Job drawing, mm, ordinate dimensions from the low corner. One solid piece. A direction names the side the tool comes from. Give positions to 0.01 mm unless a question says otherwise; leave off trailing zeros. Order: outer loops, then holes, each group sorted by start corner. A loop starts at its lowest first (then second) coordinate and runs counter-clockwise, first axis right, second up. Notation, with made-up numbers: (70.25, -36.5) - (101.25, -36.5) arc R32 cw to (101.25, -0.5) - close; hole circle Ø10 at (44.25, 56.25). An arc over 180 degrees is marked (long way). Use a Markdown table: item, result. Add a question column.
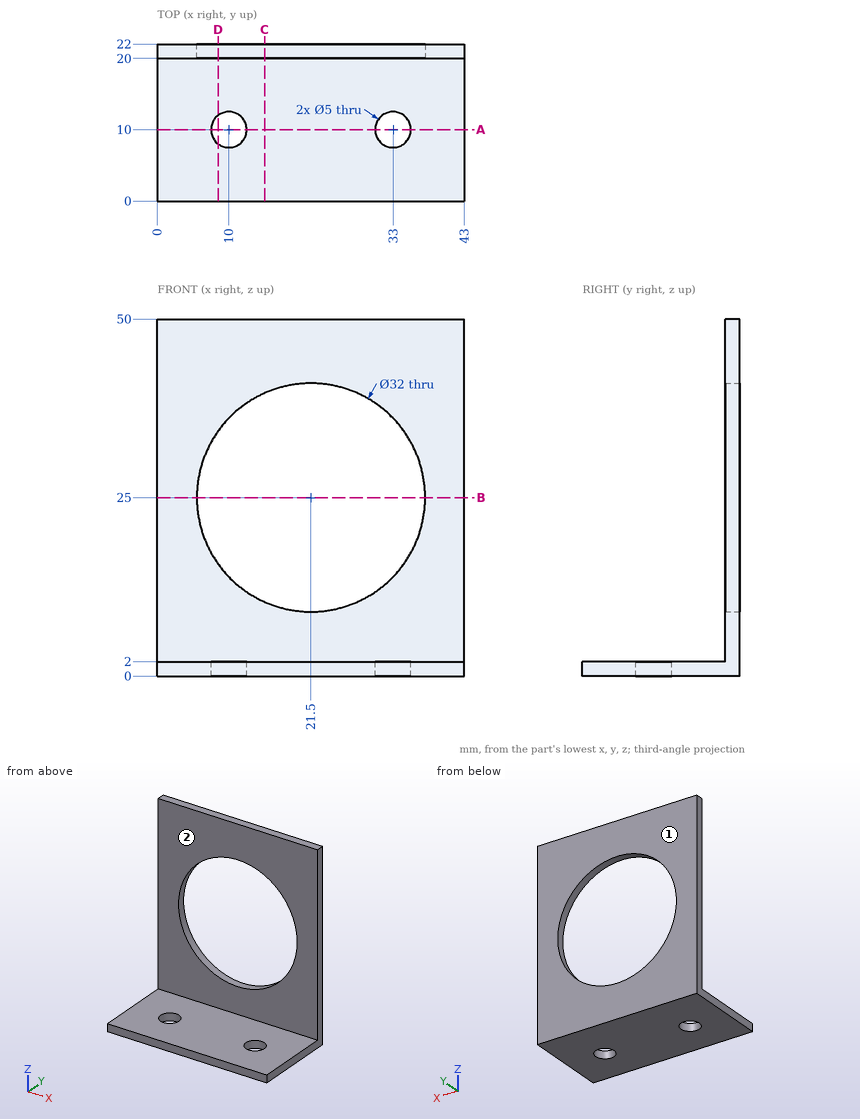
1. Tool access for the marked faces 1 and 2: list every direction of +Z, -Z, +X, -X, +Y, -Y with a clear straight run to the whole face (end or side of a thin tool).
2. Pin check, flat tips, straight feed: P1, Ø8, axis at x = 33, y = 10, coming from the +Z side; P2, Ø4.5, axis at x = 10, y = 10, coming from the -Z side. Stop position of each tip, or through.
3. Drill centre lines: probe 1 along X at (y, z) = (10, 0.6); probe 2 along Z at (x, y) = (21.5, 20.6); probe 3 along Y at (x, z) = (33, 0.7). Where is each one in solid material? Low to high. Write a range as [from, to].
4. Cut at B-B (z = 25). Write the cut outline in (x, y), plus the area to 3 significant figures.
5. Cut at C-C (x = 15). Write the cut outline in (y, z), plus the area to 3 significant figures.
6. Cut at D-D (x = 8.5). Write the cut outline in (y, z).
7. Cut at A-A (y = 10). Write the cut outline in (x, z), plus the area to 3 significant figures.
Responses:
| question | item | result |
|---|---|---|
| 1 | face 1 | +Z, -Z, +X, -X, +Y |
| 1 | face 2 | +Z, +X, -X, -Y |
| 2 | P1 | stops at z = 2 |
| 2 | P2 | passes through |
| 3 | probe 1 | x = [0, 7.5], [12.5, 30.5], [35.5, 43] |
| 3 | probe 2 | z = [0, 9], [41, 50] |
| 3 | probe 3 | y = [0, 7.5], [12.5, 22] |
| 4 | outline | (0, 20) - (5.5, 20) - (5.5, 22) - (0, 22) - close; (37.5, 20) - (43, 20) - (43, 22) - (37.5, 22) - close |
| 4 | area | 22.0 mm² |
| 5 | outline | (0, 0) - (22, 0) - (22, 10.38) - (20, 10.38) - (20, 2) - (0, 2) - close; (20, 39.62) - (22, 39.62) - (22, 50) - (20, 50) - close |
| 5 | area | 81.5 mm² |
| 6 | outline | (0, 0) - (8, 0) - (8, 2) - (0, 2) - close; (12, 0) - (22, 0) - (22, 15.67) - (20, 15.67) - (20, 2) - (12, 2) - close; (20, 34.33) - (22, 34.33) - (22, 50) - (20, 50) - close |
| 7 | outline | (0, 0) - (7.5, 0) - (7.5, 2) - (0, 2) - close; (12.5, 0) - (30.5, 0) - (30.5, 2) - (12.5, 2) - close; (35.5, 0) - (43, 0) - (43, 2) - (35.5, 2) - close |
| 7 | area | 66.0 mm² |
